from build123d import *

# Parameters (mm, degrees)
SKETCH1_R           = 3.925
BOSS_EXTRUDE1_DEPTH = 11
SKETCH2_R           = 5.084149635
BOSS_EXTRUDE2_DEPTH = 1.4
SKETCH3_R           = 2.4
CUT_EXTRUDE1_DEPTH  = 13.4
CHAMFER1_SIZE       = 0.25


with BuildPart() as part:
    # Sketch1 → Boss-Extrude1 (new body)
    with BuildSketch(Plane.XY):
        Circle(SKETCH1_R)
    extrude(amount=-BOSS_EXTRUDE1_DEPTH)

    # Sketch2 → Boss-Extrude2 (add)
    with BuildSketch(Plane.XY):
        Circle(SKETCH2_R)
    extrude(amount=BOSS_EXTRUDE2_DEPTH)

    # Sketch3 → Cut-Extrude1 (cut, through all)
    with BuildSketch(Plane.XY.offset(1.4)):
        Circle(SKETCH3_R)
    extrude(amount=-CUT_EXTRUDE1_DEPTH, mode=Mode.SUBTRACT)

    # Chamfer1
    chamfer1_edges = [part.edges().sort_by_distance(p)[0] for p in [
        (-2.4, 0, -11),
        (-2.4, 0, 1.4),
        (-3.925, 0, -11),
        (-5.084149635, 0, 0),
        (-5.084149635, 0, 1.4),
    ]]
    chamfer(chamfer1_edges, length=CHAMFER1_SIZE)


solid = part.part
The listing builds one solid part. Answer for the finished solid, in the listing's coordinates (mm). Coordinates: 2 decimals unless noted, no trailing zeros. Write each loop counter-clockwise with the first axis right and the second up, starting at its lowest first coordinate (ties: lowest second). Pieces come first, ordered by that corner, then holes. Notation, with made-up numbers: M -24.75,29 L -16.75,29 A33 cw -16.75,61 Z; hole C -21,-36 d1. An arc over 180 degrees is marked long. Put each result on its own line as item: value. Start each with the question number.
1. For a pull along X with two mould halves and no side action, classify faces 1 (the flat face through (-1, 4, 0)), 2 (the cylindrical face through (1.29, 2.024, -4.717)), 3 (the cylindrical face through (-2.893, 2.653, -5.3)) as pulls with the +X half, pulls with the -X half, needs draft (parallel to the pull), parting line crosses it, or undercut.
2. A cutting plane is placed at A-A on x = 0. Write down the section's boundary in (y, z) (3 decimals), then the cut area to 3 significant figures.
3. Consider line 1 (Y direction, x = 0, z = -6) (3 decimals); line 2 (Z direction, x = 4, y = -1.75); line 3 (X direction, y = 0.75, z = -8.75). Determine where each line is inside the solid, lowest interval first. Write a range as from..to.
4. Flat-ended cylindrical pins translate along their axes: P1, Ø4, axis at y = -1, z = -9.5, coming from the -X side (3 decimals); P2, Ø1.5, axis at y = -0.5, z = -8, coming from the +X side (3 decimals); P3, Ø1, axis at y = 2.5, z = 0, coming from the -X side (3 decimals). Find the tip coordinate at first contact, or state that the pin passes through.
5. A cutting plane is placed at C-C on z = -8.5. Write down the section's boundary in (x, y) (3 decimals).
Resolved:
1. face 1: needs draft
1. face 2: undercut
1. face 3: parting line crosses it
2. outline: M -5.084,0.25 L -4.834,0 L -3.925,0 L -3.925,-10.75 L -3.675,-11 L -2.65,-11 L -2.4,-10.75 L -2.4,1.15 L -2.65,1.4 L -4.834,1.4 L -5.084,1.15 Z; M 2.4,-10.75 L 2.65,-11 L 3.675,-11 L 3.925,-10.75 L 3.925,0 L 4.834,0 L 5.084,0.25 L 5.084,1.15 L 4.834,1.4 L 2.65,1.4 L 2.4,1.15 Z
2. area: 40.8 mm2
3. line 1: y = -3.925..-2.4, 2.4..3.925
3. line 2: z = 0..1.4
3. line 3: x = -3.85..-2.28, 2.28..3.85
4. P1: stops at x = -3.925
4. P2: stops at x = 3.925
4. P3: stops at x = -4.645
5. outline: C 0,0 d7.85; hole C 0,0 d4.8
